Part model, mm, in its own coordinate system. A direction names the side the tool comes from. Give positions to 0.01 mm unless a question says otherwise; leave off trailing zeros. Write each loop counter-clockwise with the first axis right and the second up, starting at its lowest first coordinate (ties: lowest second). Pieces come first, ordered by that corner, then holes. Notation, with made-up numbers: M -33.5,42 L -2.5,42 A14 ccw -2.5,46 Z; hole C -2.5,53 d2. An arc over 180 degrees is marked long. Answer as CSV lines item,"result". Start each with the question number.
1) Pin check, flat tips, straight feed: pin 1 Ø1.9 at (x, y) = (-354.35, 47.58) entering from -Z; pin 2 Ø1.5 at (y, z) = (52, -1.5) entering from -X; pin 3 Ø3.5 at (x, y) = (-319.71, -12.42) entering from -Z; pin 4 Ø1.5 at (x, y) = (-318.5, 67.5) entering from +Z. Stop position of each tip, or through.
2) Slice it at B-B, the plane z = -2.75. Give the cut face in (x, y), plus the area to 3 significant figures.
3) Slice it at A-A, the plane z = 1.75. Give the cut face in (x, y).
4) Tool access for faces 3 (the cylindrical face through (-352.75, 47.65, -3.9)), 4 (the cylindrical face through (-319.604, -9.623, 1.275)), 5 (the cylindrical face through (-341.97, 18.35, -6.46)): list every direction of +Z, -Z, +X, -X, +Y, -Y with a clear straight run to the whole face (end or side of a thin tool).
5) Wall check: line 1 along Y through (x, z) = (-298.5, -5.75); line 2 along X through (y, z) = (18, -5.5); line 3 along Y through (x, z) = (-302, -5.75). Give the ranges that are in metal, low to high. Write a range as from..to.
6) Mould opens along Y. For faces 1 (the flat face through (-345, -1, -7.2)), 2 (the flat face through (-321, 69, -0.5)) say: pulls with the +Y half, pulls with the -Y half, needs draft (parallel to the pull), parting line crosses it, or undercut.
```python
from build123d import *

# Parameters (mm, degrees)
SKETCH1_R           = 42.5
SKETCH1_R_2         = 1.6
SKETCH1_R_3         = 17.5
BOSS_EXTRUDE1_DEPTH = 3
BOSS_EXTRUDE3_START = 7.2
SKETCH2_R           = 42.5
SKETCH2_R_2         = 37.5
SKETCH2_R_3         = 1.6
SKETCH2_R_4         = 24.1
SKETCH2_R_5         = 21.1
BOSS_EXTRUDE3_DEPTH = 7.2
SKETCH3_R           = 2.8
CUT_EXTRUDE1_DEPTH  = 3.5
SKETCH4_R           = 37.5
SKETCH4_R_2         = 24.1
BOSS_EXTRUDE4_DEPTH = 7.2
SKETCH23_R          = 37.5
SKETCH23_R_2        = 24.1
CUT_EXTRUDE3_DEPTH  = 3
FILLET1_R           = 1.5


with BuildPart() as part:
    # Sketch1 → Boss-Extrude1 (new body)
    with BuildSketch(Plane.XY):
        with Locations((-319.708249559, 27.578631729)):
            Circle(SKETCH1_R)
        with Locations((-285.067233407, 47.578631729)):
            Circle(SKETCH1_R_2, mode=Mode.SUBTRACT)
        with Locations((-285.067233407, 7.578631729)):
            Circle(SKETCH1_R_2, mode=Mode.SUBTRACT)
        with Locations((-319.708249559, -12.421368271)):
            Circle(SKETCH1_R_2, mode=Mode.SUBTRACT)
        with Locations((-354.34926571, 7.578631729)):
            Circle(SKETCH1_R_2, mode=Mode.SUBTRACT)
        with Locations((-354.34926571, 47.578631729)):
            Circle(SKETCH1_R_2, mode=Mode.SUBTRACT)
        with Locations((-319.708249559, 67.578631729)):
            Circle(SKETCH1_R_2, mode=Mode.SUBTRACT)
        with Locations((-319.708249559, 27.578631729)):
            Circle(SKETCH1_R_3, mode=Mode.SUBTRACT)
    extrude(amount=BOSS_EXTRUDE1_DEPTH)

    # Sketch2 → Boss-Extrude3 (add)
    # profile 1 of 2: a face of its own
    with BuildSketch(Plane(origin=(0, 0, 0), x_dir=(-1, 0, 0), z_dir=(0, 0, -1)).offset(BOSS_EXTRUDE3_START)):
        with Locations((319.708249559, 27.578631729)):
            Circle(SKETCH2_R)
        with Locations((319.708249559, 27.578631729)):
            Circle(SKETCH2_R_2, mode=Mode.SUBTRACT)
        with Locations((285.067233407, 47.578631729)):
            Circle(SKETCH2_R_3, mode=Mode.SUBTRACT)
        with Locations((285.067233407, 7.578631729)):
            Circle(SKETCH2_R_3, mode=Mode.SUBTRACT)
        with Locations((354.34926571, 7.578631729)):
            Circle(SKETCH2_R_3, mode=Mode.SUBTRACT)
        with Locations((319.708249559, 67.578631729)):
            Circle(SKETCH2_R_3, mode=Mode.SUBTRACT)
        with Locations((354.34926571, 47.578631729)):
            Circle(SKETCH2_R_3, mode=Mode.SUBTRACT)
        with Locations((319.708249559, -12.421368271)):
            Circle(SKETCH2_R_3, mode=Mode.SUBTRACT)
    # profile 2 of 2: a face of its own
    with BuildSketch(Plane(origin=(0, 0, 0), x_dir=(-1, 0, 0), z_dir=(0, 0, -1)).offset(BOSS_EXTRUDE3_START)):
        with Locations(Location((319.708249559, 27.578631729, 0), (0, 0, 180))):
            Circle(SKETCH2_R_4)
        with Locations((319.708249559, 27.578631729)):
            Circle(SKETCH2_R_5, mode=Mode.SUBTRACT)
    extrude(amount=-BOSS_EXTRUDE3_DEPTH)

    # Sketch3 → Cut-Extrude1 (cut)
    with BuildSketch(Plane.XY.offset(3)):
        with Locations((-285.067233407, 47.578631729)):
            Circle(SKETCH3_R)
        with Locations((-285.067233407, 7.578631729)):
            Circle(SKETCH3_R)
        with Locations((-319.708249559, -12.421368271)):
            Circle(SKETCH3_R)
        with Locations((-354.34926571, 7.578631729)):
            Circle(SKETCH3_R)
        with Locations((-354.34926571, 47.578631729)):
            Circle(SKETCH3_R)
        with Locations((-319.708249559, 67.578631729)):
            Circle(SKETCH3_R)
    extrude(amount=-CUT_EXTRUDE1_DEPTH, mode=Mode.SUBTRACT)

    # Sketch4 → Boss-Extrude4 (add)
    with BuildSketch(Plane(origin=(0, 0, -7.2), x_dir=(-1, 0, 0), z_dir=(0, 0, -1))):
        with Locations((319.708249559, 27.578631729)):
            Circle(SKETCH4_R)
        with Locations((319.708249559, 27.578631729)):
            Circle(SKETCH4_R_2, mode=Mode.SUBTRACT)
    extrude(amount=-BOSS_EXTRUDE4_DEPTH)

    # Sketch23 → Cut-Extrude3 (cut)
    with BuildSketch(Plane(origin=(0, 0, -7.2), x_dir=(-1, 0, 0), z_dir=(0, 0, -1))):
        with Locations((319.708249559, 27.578631729)):
            Circle(SKETCH23_R)
        with Locations((319.708249559, 27.578631729)):
            Circle(SKETCH23_R_2, mode=Mode.SUBTRACT)
    extrude(amount=-CUT_EXTRUDE3_DEPTH, mode=Mode.SUBTRACT)

    # Fillet1
    fillet1_edges = [part.edges().sort_by_distance(p)[0] for p in [
        (-282.208249559, 27.578631729, -4.2),
        (-295.608249559, 27.578631729, -4.2),
    ]]
    fillet(fillet1_edges, radius=FILLET1_R)


solid = part.part
```
Found:
1,pin 1,"through"
1,pin 2,"x = -355.01"
1,pin 3,"z = -7.2"
1,pin 4,"z = -0.5"
2,outline,"C -319.71,27.58 d85; hole C -354.35,7.58 d3.2; hole C -354.35,47.58 d3.2; hole C -319.71,27.58 d42.2; hole C -319.71,-12.42 d3.2; hole C -319.71,67.58 d3.2; hole C -285.07,7.58 d3.2; hole C -285.07,47.58 d3.2"
2,area,"4,230 mm²"
3,outline,"M -357.15,7.46 A2.8 cw long -355.85,5.21 A42.5 ccw -321.01,-14.9 A2.8 cw long -318.41,-14.9 A42.5 ccw -283.57,5.21 A2.8 cw long -282.27,7.46 A42.5 ccw -282.27,47.69 A2.8 cw long -283.57,49.94 A42.5 ccw -318.41,70.06 A2.8 cw long -321.01,70.06 A42.5 ccw -355.85,49.94 A2.8 cw long -357.15,47.69 A42.5 ccw Z; hole C -319.71,27.58 d35"
4,face 3,"+Z, -Z"
4,face 4,"+Z"
4,face 5,"-Z"
5,line 1,"-9.25..-3.35, 16.13..39.03, 58.51..64.41"
5,line 2,"-361.11..-355.95, -341.84..-338.51, -300.91..-297.58, -283.47..-278.3"
5,line 3,"-11.06..-5.48, 11.23..16.11, 39.05..43.93, 60.63..66.21"
6,face 1,"needs draft"
6,face 2,"undercut"
